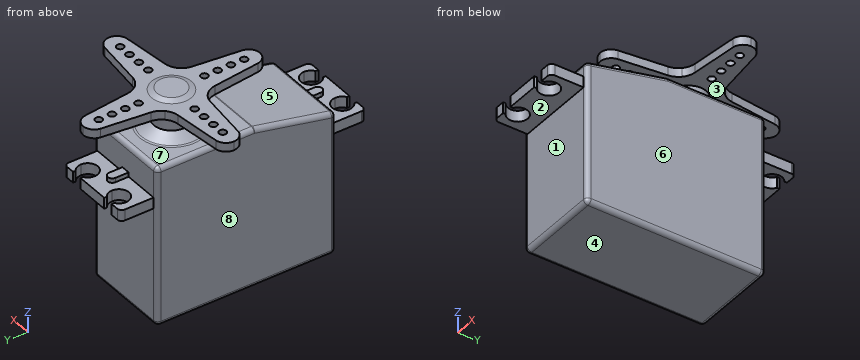
from build123d import *

# Parameters (mm, degrees)
F1_DEPTH  = 10
F0_W      = 7.5
F0_H      = 2.5
F2_DEPTH  = 9
F4_DEPTH  = 25
F5_W      = 2
F5_H      = 46.5
F6_DEPTH  = 1
F9_R      = 0.8128
F10_DEPTH = 2
F11_R     = 26.294756744
F12_DEPTH = 2
F13_R     = 0.99999


# Not quite as in the source:
# - a fillet or chamfer is up to 0.001 mm smaller than in the source, because OpenCascade refuses the exact size


with BuildPart() as f1:
    # F0 (on Right) → F1 (new body, symmetric)
    with BuildSketch(Plane.YZ):
        Polygon((-20.25, 26.6), (-20.25, 0), (20.25, 0), (20.25, 26.6), (20.25, 29.1), (20.25, 36.1), (-1.95, 36.1), (-20.25, 32.1), (-20.25, 29.1), align=None)
    extrude(amount=F1_DEPTH, both=True)

    # F0 (on Right) → F2 (join, symmetric)
    with BuildSketch(Plane.YZ):
        with Locations((-24, 27.85)):
            Rectangle(F0_W, F0_H)
        with Locations((24, 27.85)):
            Rectangle(F0_W, F0_H)
    extrude(amount=F2_DEPTH, both=True)

    # F3 (on face) → F4 (cut)
    with BuildSketch(Plane.XY.offset(29.1)):
        with BuildLine():
            ThreePointArc((-3.8, -27.1532866311), (-3.0299111695, -26.336853256), (-2.75, -25.25))
            ThreePointArc((-2.75, -25.25), (-6.086853256, -23.2799111695), (-6.2, -27.1532866311))
            ThreePointArc((-6.2, -27.1532866311), (-5, -27.5), (-3.8, -27.1532866311))
        make_face()
        with BuildLine():
            ThreePointArc((-3.8, -27.1532866311), (-5, -27.5), (-6.2, -27.1532866311))
            Line((-6.2, -27.1532866311), (-6.2, -27.75))
            Line((-6.2, -27.75), (-3.8, -27.75))
            Line((-3.8, -27.75), (-3.8, -27.1532866311))
        make_face()
        with BuildLine():
            Line((-3.8, 27.75), (-6.2, 27.75))
            Line((-6.2, 27.75), (-6.2, 27.1532866311))
            ThreePointArc((-6.2, 27.1532866311), (-5, 27.5), (-3.8, 27.1532866311))
            Line((-3.8, 27.1532866311), (-3.8, 27.75))
        make_face()
        with BuildLine():
            ThreePointArc((-3.8, 27.1532866311), (-5, 27.5), (-6.2, 27.1532866311))
            ThreePointArc((-6.2, 27.1532866311), (-6.086853256, 23.2799111695), (-2.75, 25.25))
            ThreePointArc((-2.75, 25.25), (-3.0299111695, 26.336853256), (-3.8, 27.1532866311))
        make_face()
        with BuildLine():
            Line((3.8, -27.1532866311), (3.8, -27.75))
            Line((3.8, -27.75), (6.2, -27.75))
            Line((6.2, -27.75), (6.2, -27.1532866311))
            ThreePointArc((6.2, -27.1532866311), (5, -27.5), (3.8, -27.1532866311))
        make_face()
        with BuildLine():
            ThreePointArc((7.25, -25.25), (3.913146744, -23.2799111695), (3.8, -27.1532866311))
            ThreePointArc((3.8, -27.1532866311), (5, -27.5), (6.2, -27.1532866311))
            ThreePointArc((6.2, -27.1532866311), (6.9700888305, -26.336853256), (7.25, -25.25))
        make_face()
        with BuildLine():
            Line((6.2, 27.75), (3.8, 27.75))
            Line((3.8, 27.75), (3.8, 27.1532866311))
            ThreePointArc((3.8, 27.1532866311), (5, 27.5), (6.2, 27.1532866311))
            Line((6.2, 27.1532866311), (6.2, 27.75))
        make_face()
        with BuildLine():
            ThreePointArc((6.2, 27.1532866311), (5, 27.5), (3.8, 27.1532866311))
            ThreePointArc((3.8, 27.1532866311), (3.913146744, 23.2799111695), (7.25, 25.25))
            ThreePointArc((7.25, 25.25), (6.9700888305, 26.336853256), (6.2, 27.1532866311))
        make_face()
    extrude(amount=-F4_DEPTH, mode=Mode.SUBTRACT)

    # F5 (on face) → F6 (join)
    with BuildSketch(Plane.XY.offset(29.1)):
        Rectangle(F5_W, F5_H)
        with BuildLine():
            Line((-1, 23.25), (1, 23.25))
            ThreePointArc((1, 23.25), (0, 24.25), (-1, 23.25))
        make_face()
        with BuildLine():
            ThreePointArc((-1, -23.25), (0, -24.25), (1, -23.25))
            Line((1, -23.25), (-1, -23.25))
        make_face()
    extrude(amount=F6_DEPTH)

    # F7 (on Right) → F8 (revolve)
    with BuildSketch(Plane.YZ):
        Polygon((9.85, 36.1), (16.85, 36.1), (13.85, 37.6), (13.85, 42.1), (29.85, 42.1), (29.85, 44.1), (14.35, 44.1), (13.1, 44.6), (9.85, 44.6), align=None)
    revolve(axis=Axis((0, 9.85, 38.956922479), (0, 0, -1)))

    # F9 (on face) → F10 (cut, through all)
    with BuildSketch(Plane.XY.offset(44.1)):
        with Locations((0, 17.3)):
            Circle(F9_R)
        with Locations((0, 20.3)):
            Circle(F9_R)
        with Locations((0, 23.3)):
            Circle(F9_R)
        with Locations((0, 26.3)):
            Circle(F9_R)
        with Locations((-16.45, 9.85)):
            Circle(F9_R)
        with Locations((-13.45, 9.85)):
            Circle(F9_R)
        with Locations((-10.45, 9.85)):
            Circle(F9_R)
        with Locations((-7.45, 9.85)):
            Circle(F9_R)
        with Locations((0, -6.6)):
            Circle(F9_R)
        with Locations((0, -3.6)):
            Circle(F9_R)
        with Locations((0, -0.6)):
            Circle(F9_R)
        with Locations((0, 2.4)):
            Circle(F9_R)
        with Locations((16.45, 9.85)):
            Circle(F9_R)
        with Locations((13.45, 9.85)):
            Circle(F9_R)
        with Locations((10.45, 9.85)):
            Circle(F9_R)
        with Locations((7.45, 9.85)):
            Circle(F9_R)
    extrude(amount=-F10_DEPTH, mode=Mode.SUBTRACT)

    # F11 (on face) → F12 (cut, through all)
    with BuildSketch(Plane.XY.offset(44.1)):
        with Locations((0, 9.85)):
            Circle(F11_R)
        with BuildLine():
            ThreePointArc((-4.8436814511, 14.6936814511), (-4.0616110554, 15.7958081166), (-3.6873277698, 17.0943570425))
            Line((-3.6873277698, 17.0943570425), (-2.5, 27.6162423281))
            ThreePointArc((-2.5, 27.6162423281), (-1.6762811024, 29.2102108544), (0, 29.85))
            ThreePointArc((0, 29.85), (1.6762811024, 29.2102108544), (2.5, 27.6162423281))
            Line((2.5, 27.6162423281), (3.6873277698, 17.0943570425))
            ThreePointArc((3.6873277698, 17.0943570425), (4.0616110554, 15.7958081166), (4.8436814511, 14.6936814511))
            ThreePointArc((4.8436814511, 14.6936814511), (5.9458081166, 13.9116110554), (7.2443570425, 13.5373277698))
            Line((7.2443570425, 13.5373277698), (17.7662423281, 12.35))
            ThreePointArc((17.7662423281, 12.35), (19.3602108544, 11.5262811024), (20, 9.85))
            ThreePointArc((20, 9.85), (19.3602108544, 8.1737188976), (17.7662423281, 7.35))
            Line((17.7662423281, 7.35), (7.2443570425, 6.1626722302))
            ThreePointArc((7.2443570425, 6.1626722302), (5.9458081166, 5.7883889446), (4.8436814511, 5.0063185489))
            ThreePointArc((4.8436814511, 5.0063185489), (4.0616110554, 3.9041918834), (3.6873277698, 2.6056429575))
            Line((3.6873277698, 2.6056429575), (2.5, -7.9162423281))
            ThreePointArc((2.5, -7.9162423281), (1.6762811024, -9.5102108544), (0, -10.15))
            ThreePointArc((0, -10.15), (-1.6762811024, -9.5102108544), (-2.5, -7.9162423281))
            Line((-2.5, -7.9162423281), (-3.6873277698, 2.6056429575))
            ThreePointArc((-3.6873277698, 2.6056429575), (-4.0616110554, 3.9041918834), (-4.8436814511, 5.0063185489))
            ThreePointArc((-4.8436814511, 5.0063185489), (-5.9458081166, 5.7883889446), (-7.2443570425, 6.1626722302))
            Line((-7.2443570425, 6.1626722302), (-17.7662423281, 7.35))
            ThreePointArc((-17.7662423281, 7.35), (-19.3602108544, 8.1737188976), (-20, 9.85))
            ThreePointArc((-20, 9.85), (-19.3602108544, 11.5262811024), (-17.7662423281, 12.35))
            Line((-17.7662423281, 12.35), (-7.2443570425, 13.5373277698))
            ThreePointArc((-7.2443570425, 13.5373277698), (-5.9458081166, 13.9116110554), (-4.8436814511, 14.6936814511))
        make_face(mode=Mode.SUBTRACT)
    extrude(amount=-F12_DEPTH, mode=Mode.SUBTRACT)

    # F13 (radius 1 in the source; OpenCascade refuses exactly that, so slightly less here)
    f13_edges = [f1.edges().sort_by_distance(p)[0] for p in [
        (10, -20.25, 16.05),
        (10, 0, 0),
        (10, 20.25, 18.05),
        (10, 9.15, 36.1),
        (10, -11.1, 34.1),
        (-10, 0, 0),
        (-10, 20.25, 18.05),
        (-10, 9.15, 36.1),
        (-10, -11.1, 34.1),
        (-10, -20.25, 16.05),
        (0, -20.25, 0),
        (0, 20.25, 0),
        (0, -1.95, 36.1),
        (0, -20.25, 32.1),
        (0, 20.25, 36.1),
        (0, 2.85, 36.1),
        (9, -27.75, 27.85),
        (-9, -27.75, 27.85),
        (9, 27.75, 27.85),
        (-9, 27.75, 27.85),
    ]]
    fillet(f13_edges, radius=F13_R)


solid = f1.part
Design review of the part built by this model. Coordinates are the model's own, in mm. Face numbers are marked on the shaded views. A direction names the side the tool comes from. Coordinates: 2 decimals unless noted, no trailing zeros. Order: outer loops, then holes, each group sorted by start corner. A loop starts at its lowest first (then second) coordinate and runs counter-clockwise, first axis right, second up.
Item 1: For the marked faces 4, 5, 6, 7 and 8, list the 3-axis set-ups (+Z, -Z, +X, -X, +Y, -Y) from which the entire face can be reached by the end or side of a thin tool; tool diameter is ignored.
Item 2: Take a section at B-B, the plane y = -0.6. Write out the cut boundary in (x, z), then the cut area to 3 significant figures.
Item 3: Take a section at C-C, the plane z = 19. Write out the cut boundary in (x, y).
Item 4: Take a section at A-A, the plane x = -13.45. Write out the cut boundary in (y, z), then the cut area to 3 significant figures.
Item 5: For pin 1 Ø17 at (y, z) = (-1, 12.5) entering from +X; pin 2 Ø1.9 at (x, y) = (-10.45, 9.85) entering from -Z; pin 3 Ø2.5 at (x, y) = (13.45, 9.85) entering from +Z, all flat-tipped, find the tip position at first contact; note any pin that passes through.
Item 6: Take a section at D-D, the plane x = 16.45. Write out the cut boundary in (y, z).
Item 7: For line 1 (X direction, y = -25, z = 28); line 2 (Z direction, x = -7, y = 8.5); line 3 (X direction, y = 4, z = 32), list the stretches that pass through material, from the lowest coordinate up.
Item 8: The part is to be moulded in two halves that separate along Z. For the marked faces 1, 2 and 3, say which applies: pulls with the +Z half, pulls with the -Z half, needs draft (parallel to the pull), parting line crosses it, or undercut.
The answers:
1. face 4: -Z, +X, -X, +Y, -Y
1. face 5: +X, -X, -Y
1. face 6: -Z, +X, +Y, -Y
1. face 7: none
1. face 8: -Z, -X, +Y, -Y
2. outline: (-10, 1) arc R1 ccw to (-9, 0) - (9, 0) arc R1 ccw to (10, 1) - (10, 35.1) arc R1 ccw to (9, 36.1) - (-9, 36.1) arc R1 ccw to (-10, 35.1) - close; (-3.33, 42.1) - (-0.81, 42.1) - (-0.81, 44.1) - (-3.33, 44.1) - close; (0.81, 42.1) - (3.33, 42.1) - (3.33, 44.1) - (0.81, 44.1) - close
2. area: 731 mm2
3. outline: (-10, -19.25) arc R1 ccw to (-9, -20.25) - (9, -20.25) arc R1 ccw to (10, -19.25) - (10, 19.25) arc R1 ccw to (9, 20.25) - (-9, 20.25) arc R1 ccw to (-10, 19.25) - close
4. outline: (6.86, 42.1) - (9.04, 42.1) - (9.04, 44.1) - (6.86, 44.1) - close; (10.66, 42.1) - (12.84, 42.1) - (12.84, 44.1) - (10.66, 44.1) - close
4. area: 8.70 mm2
5. pin 1: stops at x = 10
5. pin 2: stops at z = 0.13
5. pin 3: stops at z = 44.1
6. outline: (7.2, 42.1) - (9.04, 42.1) - (9.04, 44.1) - (7.2, 44.1) - close; (10.66, 42.1) - (12.5, 42.1) - (12.5, 44.1) - (10.66, 44.1) - close
7. line 1: x = -9 to -7.24, -2.76 to 2.76, 7.24 to 9
7. line 2: z = 0 to 36.11, 42.1 to 44.1
7. line 3: x = -10 to 10
8. face 1: needs draft
8. face 2: pulls with the -Z half
8. face 3: undercut
